from build123d import *

# Parameters (mm, degrees)
BOSS_EXTRU_1_DEPTH = 20


with BuildPart() as part:
    # Esquisse1 → Boss.-Extru.1 (new body)
    with BuildSketch(Plane(origin=(0, 0, 0), x_dir=(1, 0, 0), z_dir=(0, 1, 0))):
        Polygon((30, -47.5), (30, 47.5), (0, 47.5), (-30, 47.5), (-30, -47.5), align=None)
        with BuildLine():
            Line((-30, -37.071067812), (-30, -22.928932188))
            Line((-30, -22.928932188), (-41.035533906, -33.964466094))
            ThreePointArc((-41.035533906, -33.964466094), (-35.586582838, -32.880602337), (-32.5, -37.5))
            ThreePointArc((-32.5, -37.5), (-32.880602337, -39.413417162), (-33.964466094, -41.035533906))
            Line((-33.964466094, -41.035533906), (-30, -37.071067812))
        make_face()
        with BuildLine():
            ThreePointArc((-32.5, -37.5), (-35.586582838, -32.880602337), (-41.035533906, -33.964466094))
            Line((-41.035533906, -33.964466094), (-39.126345597, -35.873654403))
            ThreePointArc((-39.126345597, -35.873654403), (-36.619828106, -35.375077075), (-35.2, -37.5))
            ThreePointArc((-35.2, -37.5), (-35.375077075, -38.380171894), (-35.873654403, -39.126345597))
            Line((-35.873654403, -39.126345597), (-33.964466094, -41.035533906))
            ThreePointArc((-33.964466094, -41.035533906), (-32.880602337, -39.413417162), (-32.5, -37.5))
        make_face()
        with BuildLine():
            Line((-39.126345597, -35.873654403), (-41.035533906, -33.964466094))
            ThreePointArc((-41.035533906, -33.964466094), (-41.035533906, -41.035533906), (-33.964466094, -41.035533906))
            Line((-33.964466094, -41.035533906), (-35.873654403, -39.126345597))
            ThreePointArc((-35.873654403, -39.126345597), (-39.126345597, -39.126345597), (-39.126345597, -35.873654403))
        make_face()
        with BuildLine():
            ThreePointArc((42.5, -37.5), (42.119397663, -35.586582838), (41.035533906, -33.964466094))
            Line((41.035533906, -33.964466094), (39.126345597, -35.873654403))
            ThreePointArc((39.126345597, -35.873654403), (39.624922925, -36.619828106), (39.8, -37.5))
            ThreePointArc((39.8, -37.5), (38.380171894, -39.624922925), (35.873654403, -39.126345597))
            Line((35.873654403, -39.126345597), (33.964466094, -41.035533906))
            ThreePointArc((33.964466094, -41.035533906), (39.413417162, -42.119397663), (42.5, -37.5))
        make_face()
        with BuildLine():
            Line((39.126345597, -35.873654403), (41.035533906, -33.964466094))
            ThreePointArc((41.035533906, -33.964466094), (33.964466094, -33.964466094), (33.964466094, -41.035533906))
            Line((33.964466094, -41.035533906), (35.873654403, -39.126345597))
            ThreePointArc((35.873654403, -39.126345597), (35.873654403, -35.873654403), (39.126345597, -35.873654403))
        make_face()
        with BuildLine():
            Line((41.035533906, -33.964466094), (30, -22.928932188))
            Line((30, -22.928932188), (30, -37.071067812))
            Line((30, -37.071067812), (33.964466094, -41.035533906))
            ThreePointArc((33.964466094, -41.035533906), (33.964466094, -33.964466094), (41.035533906, -33.964466094))
        make_face()
        with BuildLine():
            Line((33.964466094, 41.035533906), (30, 37.071067812))
            Line((30, 37.071067812), (30, 22.928932188))
            Line((30, 22.928932188), (41.035533906, 33.964466094))
            ThreePointArc((41.035533906, 33.964466094), (33.964466094, 33.964466094), (33.964466094, 41.035533906))
        make_face()
        with BuildLine():
            ThreePointArc((42.5, 37.5), (39.413417162, 42.119397663), (33.964466094, 41.035533906))
            Line((33.964466094, 41.035533906), (35.873654403, 39.126345597))
            ThreePointArc((35.873654403, 39.126345597), (38.380171894, 39.624922925), (39.8, 37.5))
            ThreePointArc((39.8, 37.5), (39.624922925, 36.619828106), (39.126345597, 35.873654403))
            Line((39.126345597, 35.873654403), (41.035533906, 33.964466094))
            ThreePointArc((41.035533906, 33.964466094), (42.119397663, 35.586582838), (42.5, 37.5))
        make_face()
        with BuildLine():
            Line((35.873654403, 39.126345597), (33.964466094, 41.035533906))
            ThreePointArc((33.964466094, 41.035533906), (33.964466094, 33.964466094), (41.035533906, 33.964466094))
            Line((41.035533906, 33.964466094), (39.126345597, 35.873654403))
            ThreePointArc((39.126345597, 35.873654403), (35.873654403, 35.873654403), (35.873654403, 39.126345597))
        make_face()
        with BuildLine():
            Line((-30, 22.928932188), (-30, 37.071067812))
            Line((-30, 37.071067812), (-33.964466094, 41.035533906))
            ThreePointArc((-33.964466094, 41.035533906), (-32.880602337, 39.413417162), (-32.5, 37.5))
            ThreePointArc((-32.5, 37.5), (-35.586582838, 32.880602337), (-41.035533906, 33.964466094))
            Line((-41.035533906, 33.964466094), (-30, 22.928932188))
        make_face()
        with BuildLine():
            ThreePointArc((-32.5, 37.5), (-32.880602337, 39.413417162), (-33.964466094, 41.035533906))
            Line((-33.964466094, 41.035533906), (-35.873654403, 39.126345597))
            ThreePointArc((-35.873654403, 39.126345597), (-35.375077075, 38.380171894), (-35.2, 37.5))
            ThreePointArc((-35.2, 37.5), (-36.619828106, 35.375077075), (-39.126345597, 35.873654403))
            Line((-39.126345597, 35.873654403), (-41.035533906, 33.964466094))
            ThreePointArc((-41.035533906, 33.964466094), (-35.586582838, 32.880602337), (-32.5, 37.5))
        make_face()
        with BuildLine():
            Line((-35.873654403, 39.126345597), (-33.964466094, 41.035533906))
            ThreePointArc((-33.964466094, 41.035533906), (-41.035533906, 41.035533906), (-41.035533906, 33.964466094))
            Line((-41.035533906, 33.964466094), (-39.126345597, 35.873654403))
            ThreePointArc((-39.126345597, 35.873654403), (-39.126345597, 39.126345597), (-35.873654403, 39.126345597))
        make_face()
    extrude(amount=BOSS_EXTRU_1_DEPTH)


solid = part.part
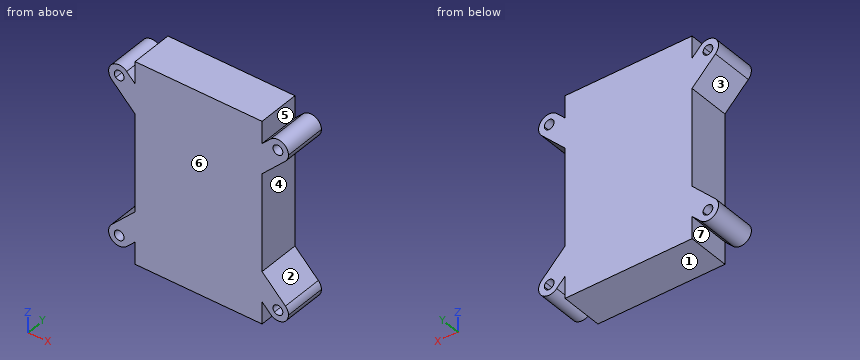
Read the model definition and answer for the solid it produces. Units are mm, in the model's axes. Face numbers are marked on the shaded views. A direction names the side the tool comes from. Round coordinates to 2 decimals unless told otherwise and drop trailing zeros. Order: outer loops, then holes, each group sorted by start corner. A loop starts at its lowest first (then second) coordinate and runs counter-clockwise, first axis right, second up. Notation, with made-up numbers: (2, 65) - (39, 65) arc R28 ccw to (39, 84) - close; hole circle Ø7 at (11.5, 26). An arc over 180 degrees is marked (long way). Use one line per item in the form item = value. Start each with the question number.
(1) The part is cut by section C-C (z = 1). Give the vertices of the cut face in (x, y).
(2) For the marked faces 1, 2 and 3, determine the directions among +Z, -Z, +X, -X, +Y, -Y from which every point of the face is accessible in a straight line to the end or side of a thin tool.
(3) The part is cut by section B-B (x = 37.5). Give the vertices of the cut face in (y, z).
(4) Determine the mould class of the marked faces 4, 5, 6 and 7 for opening direction X: +X half, -X half, draft (parallel to the pull), parting line (faces both ways), or undercut.
(5) Flat-ended cylindrical pins translate along their axes: pin 1 Ø8.5 at (y, z) = (7.5, 43.5) entering from -X; pin 2 Ø3 at (y, z) = (13.5, -42) entering from +X; pin 3 Ø2 at (x, y) = (34, 16) entering from +Z. Find the tip coordinate at first contact, or state that the pin passes through.
(6) Find the intervals of material crossed by line 1 along X through (y, z) = (8, -39.5); line 2 along X through (y, z) = (11.5, -36); line 3 along X through (y, z) = (6.25, 2), in increasing order. Write a range as from..to.
(7) The part is cut by section A-A (y = 10.5). Give the vertices of the cut face in (x, z).
Checked values:
q1.outline = (-30, 0) - (30, 0) - (30, 20) - (-30, 20) - close
q2.face_1 = -Z, +X, -X, +Y, -Y
q2.face_2 = +X, +Y, -Y
q2.face_3 = -X, +Y, -Y
q3.outline = (0, -42.5) - (20, -42.5) - (20, -39.8) - (0, -39.8) - close; (0, -35.2) - (20, -35.2) - (20, -30.43) - (0, -30.43) - close; (0, 30.43) - (20, 30.43) - (20, 35.2) - (0, 35.2) - close; (0, 39.8) - (20, 39.8) - (20, 42.5) - (0, 42.5) - close
q4.face_4 = +X half
q4.face_5 = undercut
q4.face_6 = draft
q4.face_7 = undercut
q5.pin_1 = -42.18
q5.pin_2 = 41.5
q5.pin_3 = 41.83
q6.line_1 = -42.08..-38.64, -36.36..-32.43, -30..30, 32.43..36.36, 38.64..42.08
q6.line_2 = -42.27..-39.24, -35.76..35.76, 39.24..42.27
q6.line_3 = -30..30
q7.outline = (-41.04, -33.96) arc R5 ccw to (-33.96, -41.04) - (-30, -37.07) - (-30, -47.5) - (30, -47.5) - (30, -37.07) - (33.96, -41.04) arc R5 ccw to (41.04, -33.96) - (30, -22.93) - (30, 22.93) - (41.04, 33.96) arc R5 ccw to (33.96, 41.04) - (30, 37.07) - (30, 47.5) - (-30, 47.5) - (-30, 37.07) - (-33.96, 41.04) arc R5 ccw to (-41.04, 33.96) - (-30, 22.93) - (-30, -22.93) - close; hole circle Ø4.6 at (-37.5, -37.5); hole circle Ø4.6 at (-37.5, 37.5); hole circle Ø4.6 at (37.5, -37.5); hole circle Ø4.6 at (37.5, 37.5)
